Autodesk Inventor part; units mm, degrees
ref_plane "YZ Plane" through (0, 0, 0) normal (1, 0, 0) x (0, 1, 0)
ref_plane "XZ Plane" through (0, 0, 0) normal (0, 1, 0) x (-1, 0, 0)
ref_plane "XY Plane" through (0, 0, 0) normal (0, 0, 1) x (1, 0, 0)
sketch "Sketch1" plane through (0, 0, 0) normal (0, 0, 1) x (1, 0, 0)
  line L0 (177.2398, 109.2972) -> (163.051, 103.3471)
  line L1 (323.85, -6.35) -> (323.85, 19.05)
  line L2 (323.85, -6.35) -> (292.1, -6.35)
  line L3 (292.1, -6.35) -> (292.1, 15.875)
  line L4 (292.1, -6.35) -> (323.85, -6.35)
  arc A0 (292.1, 15.875) -> (285.75, 22.225) centre (285.75, 15.875) ccw
  circle A1 centre (317.5, 0) radius 2.0955
  circle A2 centre (317.5, 12.7) radius 2.0955
  line L5 (120.65, 22.225) -> (184.15, 22.225)
  circle A3 centre (298.45, 6.35) radius 2.0955
  arc A4 (201.8633, 106.5157) -> (177.2398, 109.2972) centre (187.0626, 85.8735) ccw
  circle A5 centre (187.9687, 91.7095) radius 11.1125
  line L6 (260.35, 28.575) -> (260.35, 38.1)
  line L7 (260.35, 38.1) -> (234.95, 38.1)
  line L8 (234.95, 38.1) -> (234.95, 28.575)
  line L9 (184.15, 22.225) -> (228.6, 22.225)
  line L10 (266.7, 22.225) -> (285.75, 22.225)
  arc A6 (228.6, 22.225) -> (234.95, 28.575) centre (228.6, 28.575) ccw
  arc A7 (260.35, 28.575) -> (266.7, 22.225) centre (266.7, 28.575) ccw
  line L11 (115.328, 32.039) -> (160.1848, 100.9551)
  line L12 (323.85, 19.05) -> (291.7679, 42.0532)
  circle A8 centre (120.65, 28.575) radius 2.0955
  circle A9 centre (165.5067, 97.4911) radius 2.0955
  arc A10 (115.328, 32.039) -> (120.65, 22.225) centre (120.65, 28.575) ccw
  arc A11 (163.051, 103.3471) -> (160.1848, 100.9551) centre (165.5067, 97.4911) ccw
  circle A12 centre (137.1826, 53.975) radius 2.0955
  line L13 (228.6, 71.8456) -> (234.95, 71.8456)
  line L14 (234.95, 71.8456) -> (234.95, 65.4956)
  line L15 (234.95, 65.4956) -> (228.6, 65.4956)
  line L16 (228.6, 65.4956) -> (228.6, 71.8456)
  line L17 (228.6, 71.8456) -> (234.95, 65.4956) construction
  line L18 (234.95, 71.8456) -> (228.6, 65.4956) construction
  line L19 (147.0693, 67.265) -> (153.4193, 67.265)
  line L20 (153.4193, 67.265) -> (153.4193, 60.915)
  line L21 (153.4193, 60.915) -> (147.0693, 60.915)
  line L22 (147.0693, 60.915) -> (147.0693, 67.265)
  line L23 (147.0693, 67.265) -> (153.4193, 60.915) construction
  line L24 (153.4193, 67.265) -> (147.0693, 60.915) construction
  circle A13 centre (212.702, 97.4911) radius 2.0955
  arc A14 (217.4543, 97.1796) -> (210.8819, 101.8921) centre (212.702, 97.4911) ccw
  line L25 (323.85, 19.05) -> (218.7724, 94.3917)
  line L26 (207.8184, 102.2458) -> (201.8633, 106.5157)
  arc A15 (207.8184, 102.2458) -> (210.8819, 101.8921) centre (209.6685, 104.8261) ccw
  arc A16 (217.4543, 97.1796) -> (218.7724, 94.3917) centre (220.6225, 96.972) ccw
  point P0 (292.1, 22.225)
  point P1 (146.05, 22.225)
  point P2 (260.35, 22.225)
  point P3 (124.6512, 46.3627)
  point P4 (148.9618, 83.7126)
  point P5 (217.0763, 95.6078)
  point P6 (209.5145, 101.0297)
  dimension "d14" = 31.75
  dimension "d15" = 28.575
  dimension "d16" = 6.35
  dimension "d18" = 4.191
  dimension "d19" = 4.191
  dimension "d29" = 4.191
  dimension "d30" = 25.4
  dimension "d32" = 22.225
  dimension "d37" = 15.875
  dimension "d38" = 6.35
  dimension "d105" = 12.7
  dimension "d106" = 12.7
  dimension "d107" = 4.191
  dimension "d108" = 6.35
  dimension "d109" = 6.35
  dimension "d110" = 6.35
  dimension "d111" = 6.35
  dimension "d113" = 4.191
  dimension "d114" = 9.525
  dimension "d115" = 3.175
extrude "Extrusion1" add sketch "Sketch1" along normal blind 1.5875
properties part number "plate_mid" material "Acetal Resin, White"
Could you check a few things on this model? Use its own coordinates, in mm. A direction names the side the tool comes from. Coordinates: 2 decimals unless noted, no trailing zeros. Write each loop counter-clockwise with the first axis right and the second up, starting at its lowest first coordinate (ties: lowest second). Pieces come first, ordered by that corner, then holes. Notation, with made-up numbers: (-22.5, 32.5) -> (13.5, 32.5) arc R17 ccw to (13.5, 50.5) -> close; hole circle Ø10 at (-30, 57). An arc over 180 degrees is marked (long way). Return JSON: item names as keys, results as strings.
(1) We'd pull the mould along X, two halves only. Please class faces 1 (the cylindrical face through (198.23, 95.97, 0.78)), 2 (the flat face through (137.44, 66.01, 0.78)), 3 (the flat face through (204.883, 104.351, 0.783)): +X half, -X half, draft (parallel to the pull), parting line (faces both ways), or undercut.
Numbers:
{"face 1": "undercut", "face 2": "-X half", "face 3": "+X half"}
(2) Imagine slicing it at B-B, the plane x = 317.5. Please give me the cut outline in (y, z), then the cut area to 3 significant figures.
Numbers:
{"outline": "(-6.35, 0) -> (-2.1, 0) -> (-2.1, 1.59) -> (-6.35, 1.59) -> close; (2.1, 0) -> (10.6, 0) -> (10.6, 1.59) -> (2.1, 1.59) -> close; (14.8, 0) -> (23.6, 0) -> (23.6, 1.59) -> (14.8, 1.59) -> close", "area": "34.2 mm2"}
(3) Imagine slicing it at A-A, the plane y = 0. Please give me the cut outline in (x, z).
Numbers:
{"outline": "(292.1, 0) -> (315.4, 0) -> (315.4, 1.59) -> (292.1, 1.59) -> close; (319.6, 0) -> (323.85, 0) -> (323.85, 1.59) -> (319.6, 1.59) -> close"}
(4) I'm going to push flat-ended pins straight in: pin 1 (4 mm diameter, centred on x = 298.45, y = 6.35, fed in from +Z); pin 2 (5 mm diameter, centred on x = 191, y = 61.5, fed in from -Z); pin 3 (0.8 mm diameter, centred on y = 70, z = 0.5, fed in from +X); pin 4 (0.8 mm diameter, centred on y = 68, z = 0.5, fed in from -X). Where does each tip first touch, or does it pass through?
Numbers:
{"pin 1": "passes through", "pin 2": "stops at z = 0", "pin 3": "stops at x = 253.35", "pin 4": "stops at x = 138.47"}
(5) Imagine slicing it at C-C, the plane z = 0.3. Count the separate pieces of the cut face and the enclosed holes in it, then the cut area to 3 significant figures.
Numbers:
{"separate pieces": "1", "enclosed holes": "10", "area": "10,500 mm2"}
(6) Imagine slicing it at D-D, the plane y = 46.5. Please give me the cut outline in (x, z), then the cut area to 3 significant figures.
Numbers:
{"outline": "(124.74, 0) -> (285.57, 0) -> (285.57, 1.59) -> (124.74, 1.59) -> close", "area": "255 mm2"}
(7) I need wall thicknesses on L1, parallel to X at y = 6.5, z = 0.2; L2, parallel to X at y = 66, z = 0.3; L3, parallel to X at y = 30, z = 0.1. Which ranges of each line are inside material? Lowest first, please.
Numbers:
{"L1": "x = 292.1 to 296.36, 300.54 to 323.85", "L2": "x = 137.43 to 147.07, 153.42 to 228.6, 234.95 to 258.37", "L3": "x = 114.46 to 119.11, 122.19 to 234.95, 260.35 to 308.58"}
(8) Which directions (+Z, -Z, +X, -X, +Y, -Y) give clear straight access to the entire face, cutting with the end or side of a thin tool? Please do faces 4 (the cylindrical face through (262.26, 24.036, 0.783)), 5 (the cylindrical face through (300.386, 7.153, 0.783)).
Numbers:
{"face 4": "+Z, -Z, -Y", "face 5": "+Z, -Z"}
